```python
from build123d import *

# Parameters (mm, degrees)
F0_W     = 588.878934
F0_H     = 296.51298
F0_R     = 76.2
F1_DEPTH = 254
F2_SIZE  = 25.4


with BuildPart() as f1:
    # F0 (on Top) → F1 (new body)
    with BuildSketch(Plane.XY):
        Rectangle(F0_W, F0_H)
        Circle(F0_R, mode=Mode.SUBTRACT)
    extrude(amount=F1_DEPTH)

    # F2
    f2_edges = [f1.edges().sort_by_distance(p)[0] for p in [
        (0, -148.25649, 254),
        (294.439467, 0, 254),
        (0, 148.25649, 254),
        (-294.439467, 0, 254),
        (294.439467, 148.25649, 127),
        (294.439467, -148.25649, 127),
        (-294.439467, -148.25649, 127),
        (-294.439467, 148.25649, 127),
        (0, 148.25649, 0),
        (294.439467, 0, 0),
        (0, -148.25649, 0),
        (-294.439467, 0, 0),
    ]]
    chamfer(f2_edges, length=F2_SIZE)


solid = f1.part
```
Source: CAD feature listing. Evaluate the final solid. Frame: model axes, mm. Give positions to 0.01 mm unless a question says otherwise; leave off trailing zeros. Order: outer loops, then holes, each group sorted by start corner. A loop starts at its lowest first (then second) coordinate and runs counter-clockwise, first axis right, second up.
(1) Pull-direction query (X, two-part tool) for faces 1 (the face through (-60.47, -46.367, 125.222)), 2 (the face through (-3.767, -135.379, 12.522)), 3 (the face through (281.56, -1.72, 241.48)); classes: +X half, -X half, draft (parallel to the pull), parting line (faces both ways), or undercut.
(2) Section query A-A (y = 0). Return the cut outline in (x, z), plus the area to 3 significant figures.
(3) Section query B-B (x = 0). Return the cut outline in (y, z), plus the area to 3 significant figures.
(4) Section query D-D (x = -244.5). Return the cut outline in (y, z).
(5) Material intervals for line 1 along X through (y, z) = (-2.5, 203); line 2 along Y through (x, z) = (0, 53.5); line 3 along Y through (x, z) = (47, 46), sorted ascending.
(6) Section query C-C (z = 83). Return the cut outline in (x, y).
Outcome:
1. face 1: undercut
1. face 2: draft
1. face 3: +X half
2. outline: (-294.44, 25.4) - (-269.04, 0) - (-76.2, 0) - (-76.2, 254) - (-269.04, 254) - (-294.44, 228.6) - close; (76.2, 0) - (269.04, 0) - (294.44, 25.4) - (294.44, 228.6) - (269.04, 254) - (76.2, 254) - close
2. area: 110,000 mm2
3. outline: (-148.26, 25.4) - (-122.86, 0) - (-76.2, 0) - (-76.2, 254) - (-122.86, 254) - (-148.26, 228.6) - close; (76.2, 0) - (122.86, 0) - (148.26, 25.4) - (148.26, 228.6) - (122.86, 254) - (76.2, 254) - close
3. area: 35,300 mm2
4. outline: (-148.26, 25.4) - (-122.86, 0) - (122.86, 0) - (148.26, 25.4) - (148.26, 228.6) - (122.86, 254) - (-122.86, 254) - (-148.26, 228.6) - close
5. line 1: x = -294.44 to -76.16, 76.16 to 294.44
5. line 2: y = -148.26 to -76.2, 76.2 to 148.26
5. line 3: y = -148.26 to -59.98, 59.98 to 148.26
6. outline: (-294.44, -122.86) - (-269.04, -148.26) - (269.04, -148.26) - (294.44, -122.86) - (294.44, 122.86) - (269.04, 148.26) - (-269.04, 148.26) - (-294.44, 122.86) - close; hole circle Ø152.4 at (0, 0)
